Geometry check sheet. Reference: the model listing, model coordinates, mm. A direction names the side the tool comes from. Coordinates: 2 decimals unless noted, no trailing zeros. Order: outer loops, then holes, each group sorted by start corner. A loop starts at its lowest first (then second) coordinate and runs counter-clockwise, first axis right, second up. Notation, with made-up numbers: (-25.5, 7) - (7.5, 7) arc R15 cw to (7.5, 29) - close; hole circle Ø7 at (-2.75, 41.25). An arc over 180 degrees is marked (long way). Use CSV: the item, a comma, the result in double quotes. Start each with the question number.
1) Sectioned sample at A-A, the plane x = 15.25. Record the cut outline in (y, z), and give its area (3 significant figures).
2) Draft check along X on faces 5 (the flat face through (-5, 0, -17)), 6 (the cylindrical face through (-0.8, 14.8, 0.9)), 7 (the cylindrical face through (6.9, 0.57, 0.94)). Enter one of: released by +X, released by -X, zero draft, split by the parting line, or undercut.
3) Sectioned sample at B-B, the plane z = 3.5. Record the cut outline in (x, y), and give its area (3 significant figures).
4) Tool access check on faces 1 (the cylindrical face through (13.44, 0.6, -5.57)), 2 (the flat face through (13, 8, -5)), 3 (the cylindrical face through (1.95, 7.25, -18.7)), 4 (the cylindrical face through (13.44, 16.13, -5.6)). Record the directions out of +Z, -Z, +X, -X, +Y, -Y that give a thin tool (end or side, any length) a straight path to the whole face; none if there is none.
5) Sectioned sample at D-D, the plane z = -12.5. Record the cut outline in (x, y).
6) Sectioned sample at C-C, the plane y = 2.75. Record the cut outline in (x, z).
7) Thickness scan on probe 1 along Y at (x, z) = (0.25, -1); probe 2 along X at (y, z) = (8.5, 2.5); probe 3 along X at (y, z) = (7.75, -12.5). Record the ranges inside material, lowest first. Write a range as [from, to].
8) Depth check by flat-ended pin: P1, Ø10, axis at y = 11.5, z = -1, coming from the +X side; P2, Ø2.5, axis at y = 6, z = 1, coming from the +X side; P3, Ø3, axis at y = 5, z = -2, coming from the +X side; P4, Ø4, axis at x = 11.5, y = 9, coming from the +Z side. Enter the tip coordinate at first touch or a pass-through.
from build123d import *

# Parameters (mm, degrees)
SKETCH1_W           = 15
SKETCH1_H           = 10
SKETCH1_H_2         = 15
SKETCH1_W_2         = 10
BOSS_EXTRUDE1_DEPTH = 16.7
SKETCH2_R           = 6.5
CUT_EXTRUDE1_DEPTH  = 8.3
SKETCH3_R           = 6.5
CUT_EXTRUDE2_DEPTH  = 8.3
SKETCH4_R           = 6.5
CUT_EXTRUDE3_DEPTH  = 14.7
FILLET8_R           = 2


with BuildPart() as part:
    # Sketch1 → Boss-Extrude1 (new body)
    with BuildSketch(Plane(origin=(0, 0, 0), x_dir=(1, 0, 0), z_dir=(0, 1, 0))):
        Rectangle(SKETCH1_W, SKETCH1_H)
        with Locations((0, 12.5)):
            Rectangle(SKETCH1_W, SKETCH1_H_2)
        with Locations((12.5, 12.5)):
            Rectangle(SKETCH1_W_2, SKETCH1_H_2)
    extrude(amount=BOSS_EXTRUDE1_DEPTH)

    # Sketch2 → Cut-Extrude1 (cut)
    with BuildSketch(Plane.XY.offset(5)):
        with Locations((0, 8.35)):
            Circle(SKETCH2_R)
    extrude(amount=-CUT_EXTRUDE1_DEPTH, mode=Mode.SUBTRACT)

    # Sketch3 → Cut-Extrude2 (cut)
    with BuildSketch(Plane(origin=(17.5, 0, 0), x_dir=(0, 0, -1), z_dir=(1, 0, 0))):
        with Locations((12.5, 8.35)):
            Circle(SKETCH3_R)
    extrude(amount=-CUT_EXTRUDE2_DEPTH, mode=Mode.SUBTRACT)

    # Sketch4 → Cut-Extrude3 (cut)
    with BuildSketch(Plane.XZ):
        with Locations(Location((0, -12.5, 0), (0, 0, 270))):
            Circle(SKETCH4_R)
    extrude(amount=-CUT_EXTRUDE3_DEPTH, mode=Mode.SUBTRACT)

    # Fillet8
    # the kernel refuses this fillet: 2 mm, written as the material it adds along each edge
    with BuildSketch(Plane(origin=(7.5, 0, -5), x_dir=(0, 0, 1), z_dir=(0, 1, 0))) as fillet8_piece_1:
        with BuildLine():
            CenterArc((FILLET8_R, FILLET8_R), FILLET8_R, 180, 90)
            Line((0, FILLET8_R), (0, 0))
            Line((0, 0), (FILLET8_R, 0))
        make_face()
    extrude(amount=16.7)
    # the kernel refuses this fillet: 2 mm, written as the material it takes off along each edge
    with BuildSketch(Plane(origin=(-5.5, 2, -18), x_dir=(0, 0, -1), z_dir=(-1, 0, 0))) as fillet8_2_piece_1_section:
        Polygon((0, 0), (FILLET8_R, 0), (FILLET8_R, FILLET8_R), (0, FILLET8_R), align=None)
    fillet8_2_piece_1 = extrude(amount=FILLET8_R, mode=Mode.PRIVATE)
    fillet8_2_piece_1 = fillet8_2_piece_1 - Plane(origin=(-5.5, 2, -18), x_dir=(0, 0.7071067811865475, 0.7071067811865475), z_dir=(-1, 0, 0)) * Sphere(FILLET8_R, mode=Mode.PRIVATE)
    add(fillet8_2_piece_1, mode=Mode.SUBTRACT)
    with BuildSketch(Plane(origin=(-5.5, 14.7, -18), x_dir=(0, 1, 0), z_dir=(-1, 0, 0))) as fillet8_2_piece_2_section:
        Polygon((0, 0), (FILLET8_R, 0), (FILLET8_R, FILLET8_R), (0, FILLET8_R), align=None)
    fillet8_2_piece_2 = extrude(amount=FILLET8_R, mode=Mode.PRIVATE)
    fillet8_2_piece_2 = fillet8_2_piece_2 - Plane(origin=(-5.5, 14.7, -18), x_dir=(0, -0.7071067811865475, 0.7071067811865475), z_dir=(-1, 0, 0)) * Sphere(FILLET8_R, mode=Mode.PRIVATE)
    add(fillet8_2_piece_2, mode=Mode.SUBTRACT)
    with BuildSketch(Plane(origin=(-7.5, 0, -18), x_dir=(0, 1, 0), z_dir=(0, 0, 1)), Plane(origin=(22.5, 16.7, -20), x_dir=(0, 0, 1), z_dir=(-1, 0, 0)), Plane(origin=(-7.5, 16.7, 10), x_dir=(0, -1, 0), z_dir=(0, 0, -1)), Plane(origin=(22.5, 0, -20), x_dir=(0, 1, 0), z_dir=(-1, 0, 0))) as fillet8_2_piece_3:
        with BuildLine():
            CenterArc((FILLET8_R, -FILLET8_R), FILLET8_R, 90, 90)
            Line((0, -FILLET8_R), (0, 0))
            Line((0, 0), (FILLET8_R, 0))
        make_face()
    extrude(amount=28, mode=Mode.SUBTRACT)
    with BuildSketch(Plane(origin=(-7.5, 2, -20), x_dir=(0, 0, 1), z_dir=(0, 1, 0))) as fillet8_2_piece_4:
        with BuildLine():
            CenterArc((FILLET8_R, FILLET8_R), FILLET8_R, 180, 90)
            Line((0, FILLET8_R), (0, 0))
            Line((0, 0), (FILLET8_R, 0))
        make_face()
    extrude(amount=12.7, mode=Mode.SUBTRACT)
    # the kernel refuses this fillet: 2 mm, written as the material it takes off along each edge
    with BuildSketch(Plane(origin=(7.5, 16.7, 10), x_dir=(-1, 0, 0), z_dir=(0, 0, -1)), Plane(origin=(9.5, 16.7, -5), x_dir=(0, 0, -1), z_dir=(1, 0, 0)), Plane(origin=(7.5, 0, -3), x_dir=(-1, 0, 0), z_dir=(0, 0, 1))) as fillet8_3_piece_1:
        with BuildLine():
            CenterArc((FILLET8_R, -FILLET8_R), FILLET8_R, 90, 90)
            Line((0, -FILLET8_R), (0, 0))
            Line((0, 0), (FILLET8_R, 0))
        make_face()
    extrude(amount=13, mode=Mode.SUBTRACT)
    with BuildSketch(Plane(origin=(9.5, 0, -5), x_dir=(0, 0, -1), z_dir=(1, 0, 0))) as fillet8_3_piece_2:
        with BuildLine():
            CenterArc((FILLET8_R, FILLET8_R), FILLET8_R, 180, 90)
            Line((0, FILLET8_R), (0, 0))
            Line((0, 0), (FILLET8_R, 0))
        make_face()
    extrude(amount=13, mode=Mode.SUBTRACT)
    with BuildSketch(Plane(origin=(9.5, 0, -3), x_dir=(-1, 0, 0), z_dir=(0, 0, 1))) as fillet8_3_piece_3:
        with BuildLine():
            CenterArc((2 + FILLET8_R, -FILLET8_R), FILLET8_R, 90, 90)
            Line((2, -FILLET8_R), (2, 0))
            Line((2, 0), (2 + FILLET8_R, 0))
        make_face()
    revolve(axis=Axis((9.5, 0, -3), (0, -1, 0)), revolution_arc=90, mode=Mode.SUBTRACT)
    with BuildSketch(Plane(origin=(9.5, 16.7, -3), x_dir=(-1, 0, 0), z_dir=(0, 0, 1))) as fillet8_3_piece_4:
        with BuildLine():
            CenterArc((2 + FILLET8_R, FILLET8_R), FILLET8_R, 180, 90)
            Line((2, FILLET8_R), (2, 0))
            Line((2, 0), (2 + FILLET8_R, 0))
        make_face()
    revolve(axis=Axis((9.5, 16.7, -3), (0, -1, 0)), revolution_arc=90, mode=Mode.SUBTRACT)


solid = part.part
Evaluation:
1,outline,"(0, -18) arc R2 ccw to (2, -20) - (14.7, -20) arc R2 ccw to (16.7, -18) - (16.7, -7) arc R2 ccw to (14.7, -5) - (2, -5) arc R2 ccw to (0, -7) - close; hole circle Ø13 at (8.35, -12.5)"
1,area,"114 mm²"
2,face 5,"zero draft"
2,face 6,"undercut"
2,face 7,"released by +X"
3,outline,"(-7.5, 2) arc R2 ccw to (-5.5, 0) - (5.5, 0) arc R2 ccw to (7.5, 2) - (7.5, 14.7) arc R2 ccw to (5.5, 16.7) - (-5.5, 16.7) arc R2 ccw to (-7.5, 14.7) - close; hole circle Ø13 at (0, 8.35)"
3,area,"114 mm²"
4,face 1,"+Z, +X, -Y"
4,face 2,"+Z, +X, +Y, -Y"
4,face 3,"-Y"
4,face 4,"+Z, +X, +Y"
5,outline,"(-7.5, 2) arc R2 ccw to (-6.5, 0.27) - (-6.5, 14.7) - (6.5, 14.7) - (6.5, 0) - (17.5, 0) - (17.5, 1.85) - (9.2, 1.85) - (9.2, 14.85) - (17.5, 14.85) - (17.5, 16.7) - (-5.5, 16.7) arc R2 ccw to (-7.5, 14.7) - close"
6,outline,"(-7.5, -18) arc R2 ccw to (-5.5, -20) - (17.5, -20) - (17.5, -15.8) - (9.2, -15.8) - (9.2, -9.2) - (17.5, -9.2) - (17.5, -5) - (9.5, -5) arc R2 cw to (7.5, -3) - (7.5, 5) - (3.3, 5) - (3.3, -3.3) - (-3.3, -3.3) - (-3.3, 5) - (-7.5, 5) - close; hole circle Ø13 at (0, -12.5)"
7,probe 1,"[0, 1.85], [14.85, 16.7]"
7,probe 2,"[-7.5, -6.5], [6.5, 7.5]"
7,probe 3,"[-7.5, -6.5], [6.5, 9.2]"
8,P1,"x = 17.5"
8,P2,"x = 7.5"
8,P3,"x = 7.56"
8,P4,"z = -5"
